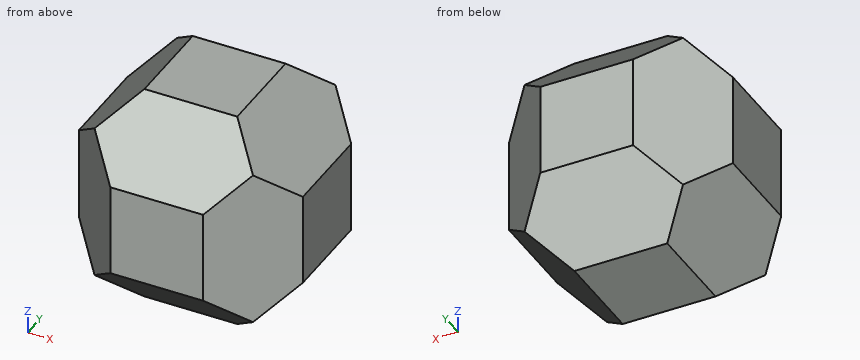
from build123d import *

# Parameters (mm, degrees)
F0_W     = 203.2
F0_H     = 203.2
F1_DEPTH = 101.6
F3_DEPTH = 203.2
F5_DEPTH = 101.6
F7_DEPTH = 101.6


with BuildPart() as f1:
    # F0 (on Front) → F1 (new body, symmetric)
    with BuildSketch(Plane.XZ):
        Rectangle(F0_W, F0_H)
    extrude(amount=F1_DEPTH, both=True)

    # F2 (on face) → F3 (cut)
    with BuildSketch(Plane.XY.offset(101.6)):
        Polygon((-101.6, 42.084098), (-42.084098, 101.6), (-101.6, 101.6), align=None)
        Polygon((101.6, 101.6), (42.084098, 101.6), (101.6, 42.084098), align=None)
        Polygon((101.6, -101.6), (101.6, -42.084098), (42.084098, -101.6), align=None)
        Polygon((-42.084098, -101.6), (-101.6, -42.084098), (-101.6, -101.6), align=None)
    extrude(amount=-F3_DEPTH, mode=Mode.SUBTRACT)

    # F4 (on Front) → F5 (cut, symmetric)
    with BuildSketch(Plane.XZ):
        Polygon((-101.6, 42.084098), (-42.084098, 101.6), (-101.6, 101.6), align=None)
        Polygon((-101.6, -101.6), (-42.084098, -101.6), (-101.6, -42.084098), align=None)
        Polygon((101.6, -101.6), (101.6, -42.084098), (42.084098, -101.6), align=None)
        Polygon((101.6, 101.6), (42.084098, 101.6), (101.6, 42.084098), align=None)
    extrude(amount=F5_DEPTH, both=True, mode=Mode.SUBTRACT)

    # F6 (on Right) → F7 (cut, symmetric)
    with BuildSketch(Plane.YZ):
        Polygon((101.6, 101.6), (42.084098, 101.6), (101.6, 42.084098), align=None)
        Polygon((101.6, -101.6), (101.6, -42.084098), (42.084098, -101.6), align=None)
        Polygon((-101.6, -101.6), (-42.084098, -101.6), (-101.6, -42.084098), align=None)
        Polygon((-101.6, 42.084098), (-42.084098, 101.6), (-101.6, 101.6), align=None)
    extrude(amount=F7_DEPTH, both=True, mode=Mode.SUBTRACT)


solid = f1.part
Here's how the part is built. I have some questions about the finished solid (model axes, mm). Give positions to 0.01 mm unless a question says otherwise; leave off trailing zeros. Order: outer loops, then holes, each group sorted by start corner. A loop starts at its lowest first (then second) coordinate and runs counter-clockwise, first axis right, second up. Notation, with made-up numbers: (37, 23.5) -> (95, 23.5) arc R33 cw to (95, 62.5) -> close; hole circle Ø3 at (21, 25.5). An arc over 180 degrees is marked (long way). Use a Markdown table: item, result. Add a question column.
Item 1: Imagine slicing it at C-C on z = 87. Please give me the cut outline in (x, y).
Item 2: I need wall thicknesses on line 1 (Z direction, x = -64.5, y = -24); line 2 (X direction, y = 82, z = 30.5); line 3 (Z direction, x = 58.5, y = -33.5). Which ranges of each line are inside material? Lowest first, please.
Item 3: Imagine slicing it at A-A on x = 7. Please give me the cut outline in (y, z).
Item 4: Will these pins go through, and if not, where does the flat tip stop? pin 1 (4 mm diameter, centred on y = -74.5, z = 29, fed in from -X); pin 2 (6 mm diameter, centred on x = -19.5, y = -53, fed in from -Z); pin 3 (8 mm diameter, centred on x = -2, z = -76.5, fed in from +Y).
Item 5: Imagine slicing it at D-D on y = 81. Please give me the cut outline in (x, z).
Data:
| question | item | result |
|---|---|---|
| 1 | outline | (-56.68, -56.68) -> (56.68, -56.68) -> (56.68, 56.68) -> (-56.68, 56.68) -> close |
| 2 | line 1 | z = -79.18 to 79.18 |
| 2 | line 2 | x = -61.68 to 61.68 |
| 2 | line 3 | z = -85.18 to 85.18 |
| 3 | outline | (-101.6, -42.08) -> (-42.08, -101.6) -> (42.08, -101.6) -> (101.6, -42.08) -> (101.6, 42.08) -> (42.08, 101.6) -> (-42.08, 101.6) -> (-101.6, 42.08) -> close |
| 4 | pin 1 | stops at x = -71.18 |
| 4 | pin 2 | stops at z = -93.68 |
| 4 | pin 3 | stops at y = 71.18 |
| 5 | outline | (-62.68, -62.68) -> (62.68, -62.68) -> (62.68, 62.68) -> (-62.68, 62.68) -> close |
